Here's how the part is built. I have some questions about the finished solid (model axes, mm). A direction names the side the tool comes from. Coordinates: 2 decimals unless noted, no trailing zeros. Order: outer loops, then holes, each group sorted by start corner. A loop starts at its lowest first (then second) coordinate and runs counter-clockwise, first axis right, second up.
```python
from build123d import *

# Parameters (mm, degrees)
F0_W          = 155
F0_H          = 40
F0_R          = 5
F1_DEPTH      = 25
F2_R          = 11
F3_DEPTH      = 10
F4_W          = 40
F4_H          = 25
F5_DEPTH      = 25
F6_R          = 4.25
F7_DEPTH      = 40
F9_DEPTH      = 6
F10_T4_DEPTH  = 25
F10_T10_DEPTH = 25
F10_T16_DEPTH = 25
F10_T23_DEPTH = 25
F10_T29_DEPTH = 25
F10_T35_DEPTH = 25
F10_T41_DEPTH = 25
F10_T47_DEPTH = 25
F10_T54_DEPTH = 25
F10_T60_DEPTH = 25
F10_T63_DEPTH = 50


# Not quite as in the source:
# - a fillet or chamfer that OpenCascade refuses, or shapes differently, is made with other operations: its cross-section is extruded or revolved along the edge and cut away or added


with BuildPart() as f1:
    # F0 (on Front) → F1 (new body)
    with BuildSketch(Plane.XZ):
        with Locations((-7.5, 0)):
            Rectangle(F0_W, F0_H)
        with Locations((-65, 0)):
            Circle(F0_R, mode=Mode.SUBTRACT)
        Circle(F0_R, mode=Mode.SUBTRACT)
        with Locations((55, 0)):
            Circle(F0_R, mode=Mode.SUBTRACT)
    extrude(amount=F1_DEPTH)

    # F2 (on face) → F3 (cut)
    with BuildSketch(Plane.XZ.offset(25)):
        with Locations((-65, 0)):
            Circle(F2_R)
        Circle(F2_R)
        with Locations((55, 0)):
            Circle(F2_R)
    extrude(amount=-F3_DEPTH, mode=Mode.SUBTRACT)

    # F4 (on face) → F5 (join)
    with BuildSketch(Plane(origin=(0, 0, 0), x_dir=(-1, 0, 0), z_dir=(0, 1, 0))):
        with Locations((65, 32.5)):
            Rectangle(F4_W, F4_H)
        with Locations((65, -32.5)):
            Rectangle(F4_W, F4_H)
    extrude(amount=-F5_DEPTH)

    # F6 (on face) → F7 (cut, through all)
    with BuildSketch(Plane(origin=(-85, 0, 0), x_dir=(0, -1, 0), z_dir=(-1, 0, 0))):
        with Locations((12.5, 27.5)):
            Circle(F6_R)
        with Locations((12.5, -27.5)):
            Circle(F6_R)
    extrude(amount=-F7_DEPTH, mode=Mode.SUBTRACT)

    # F8 (on face) → F9 (cut)
    with BuildSketch(Plane.YZ.offset(-45)):
        Polygon((-8.4585481157, 34.5), (-16.5414518843, 34.5), (-20.5829037687, 27.5), (-16.5414518843, 20.5), (-8.4585481157, 20.5), (-4.4170962313, 27.5), align=None)
        Polygon((-8.4585481157, -20.5), (-16.5414518843, -20.5), (-20.5829037687, -27.5), (-16.5414518843, -34.5), (-8.4585481157, -34.5), (-4.4170962313, -27.5), align=None)
    extrude(amount=-F9_DEPTH, mode=Mode.SUBTRACT)

    # F10: fillet of radius 5 on 6 edges, made by hand


with BuildPart() as f10_tool2:
    # F10_s3 → F10_t4 (new body)
    with BuildSketch(Plane.XZ):
        with BuildLine():
            ThreePointArc((-40, 20), (-43.5355339059, 21.4644660941), (-45, 25))
            Line((-45, 25), (-45, 20))
            Line((-45, 20), (-40, 20))
        make_face()
    extrude(amount=F10_T4_DEPTH)

    split(bisect_by=Plane.XY.offset(20.5), keep=Keep.BOTTOM)

    split(bisect_by=Plane(origin=(0, -15.2206714755, 8.7876587737), x_dir=(1, 0, 0), z_dir=(0, 0.8660254038, -0.5)), keep=Keep.TOP)


with BuildPart() as f1_1:
    add(f1.part)

    # F10_t1: union F10_tool2
    add(f10_tool2.part)


with BuildPart() as f10_tool8:
    # F10_s9 → F10_t10 (new body)
    with BuildSketch(Plane.XZ):
        with BuildLine():
            ThreePointArc((-40, 20), (-43.5355339059, 21.4644660941), (-45, 25))
            Line((-45, 25), (-45, 20))
            Line((-45, 20), (-40, 20))
        make_face()
    extrude(amount=F10_T10_DEPTH)

    split(bisect_by=Plane.XY.offset(20.5), keep=Keep.TOP)

    split(bisect_by=Plane(origin=(0, -15.2206714755, 8.7876587737), x_dir=(1, 0, 0), z_dir=(0, 0.8660254038, -0.5)), keep=Keep.TOP)


with BuildPart() as f1_2:
    add(f1_1.part)

    # F10_t7: union F10_tool8
    add(f10_tool8.part)


with BuildPart() as f10_tool14:
    # F10_s15 → F10_t16 (new body)
    with BuildSketch(Plane.XZ):
        with BuildLine():
            ThreePointArc((-40, 20), (-43.5355339059, 21.4644660941), (-45, 25))
            Line((-45, 25), (-45, 20))
            Line((-45, 20), (-40, 20))
        make_face()
    extrude(amount=F10_T16_DEPTH)

    split(bisect_by=Plane(origin=(0, -3.5293285245, -2.0376587737), x_dir=(1, 0, 0), z_dir=(0, 0.8660254038, 0.5)), keep=Keep.TOP)

    split(bisect_by=Plane.XY.offset(20.5), keep=Keep.BOTTOM)

    split(bisect_by=Plane(origin=(0, -15.2206714755, 8.7876587737), x_dir=(1, 0, 0), z_dir=(0, -0.8660254038, 0.5)), keep=Keep.TOP)


with BuildPart() as f1_3:
    add(f1_2.part)

    # F10_t13: union F10_tool14
    add(f10_tool14.part)


with BuildPart() as f10_tool21:
    # F10_s22 → F10_t23 (new body)
    with BuildSketch(Plane.XZ):
        with BuildLine():
            ThreePointArc((-40, 20), (-43.5355339059, 21.4644660941), (-45, 25))
            Line((-45, 25), (-45, 20))
            Line((-45, 20), (-40, 20))
        make_face()
    extrude(amount=F10_T23_DEPTH)

    split(bisect_by=Plane(origin=(0, -3.5293285245, -2.0376587737), x_dir=(1, 0, 0), z_dir=(0, -0.8660254038, -0.5)), keep=Keep.TOP)

    split(bisect_by=Plane.XY.offset(20.5), keep=Keep.BOTTOM)


with BuildPart() as f1_4:
    add(f1_3.part)

    # F10_t20: union F10_tool21
    add(f10_tool21.part)


with BuildPart() as f10_tool27:
    # F10_s28 → F10_t29 (new body)
    with BuildSketch(Plane.XZ):
        with BuildLine():
            ThreePointArc((-40, 20), (-43.5355339059, 21.4644660941), (-45, 25))
            Line((-45, 25), (-45, 20))
            Line((-45, 20), (-40, 20))
        make_face()
    extrude(amount=F10_T29_DEPTH)

    split(bisect_by=Plane(origin=(0, -3.5293285245, -2.0376587737), x_dir=(1, 0, 0), z_dir=(0, -0.8660254038, -0.5)), keep=Keep.TOP)

    split(bisect_by=Plane.XY.offset(20.5), keep=Keep.TOP)


with BuildPart() as f1_5:
    add(f1_4.part)

    # F10_t26: union F10_tool27
    add(f10_tool27.part)


with BuildPart() as f10_tool33:
    # F10_s34 → F10_t35 (new body)
    with BuildSketch(Plane.XZ):
        with BuildLine():
            ThreePointArc((-40, -20), (-43.5355339059, -21.4644660941), (-45, -25))
            Line((-45, -25), (-45, -20))
            Line((-45, -20), (-40, -20))
        make_face()
    extrude(amount=F10_T35_DEPTH)

    split(bisect_by=Plane.XY.offset(-20.5), keep=Keep.TOP)

    split(bisect_by=Plane(origin=(0, -15.2206714755, -8.7876587737), x_dir=(1, 0, 0), z_dir=(0, 0.8660254038, 0.5)), keep=Keep.TOP)


with BuildPart() as f1_6:
    add(f1_5.part)

    # F10_t32: union F10_tool33
    add(f10_tool33.part)


with BuildPart() as f10_tool39:
    # F10_s40 → F10_t41 (new body)
    with BuildSketch(Plane.XZ):
        with BuildLine():
            ThreePointArc((-40, -20), (-43.5355339059, -21.4644660941), (-45, -25))
            Line((-45, -25), (-45, -20))
            Line((-45, -20), (-40, -20))
        make_face()
    extrude(amount=F10_T41_DEPTH)

    split(bisect_by=Plane.XY.offset(-20.5), keep=Keep.BOTTOM)

    split(bisect_by=Plane(origin=(0, -15.2206714755, -8.7876587737), x_dir=(1, 0, 0), z_dir=(0, 0.8660254038, 0.5)), keep=Keep.TOP)


with BuildPart() as f1_7:
    add(f1_6.part)

    # F10_t38: union F10_tool39
    add(f10_tool39.part)


with BuildPart() as f10_tool45:
    # F10_s46 → F10_t47 (new body)
    with BuildSketch(Plane.XZ):
        with BuildLine():
            ThreePointArc((-40, -20), (-43.5355339059, -21.4644660941), (-45, -25))
            Line((-45, -25), (-45, -20))
            Line((-45, -20), (-40, -20))
        make_face()
    extrude(amount=F10_T47_DEPTH)

    split(bisect_by=Plane.XY.offset(-20.5), keep=Keep.TOP)

    split(bisect_by=Plane(origin=(0, -3.5293285245, 2.0376587737), x_dir=(1, 0, 0), z_dir=(0, 0.8660254038, -0.5)), keep=Keep.TOP)

    split(bisect_by=Plane(origin=(0, -15.2206714755, -8.7876587737), x_dir=(1, 0, 0), z_dir=(0, -0.8660254038, -0.5)), keep=Keep.TOP)


with BuildPart() as f1_8:
    add(f1_7.part)

    # F10_t44: union F10_tool45
    add(f10_tool45.part)


with BuildPart() as f10_tool52:
    # F10_s53 → F10_t54 (new body)
    with BuildSketch(Plane.XZ):
        with BuildLine():
            ThreePointArc((-40, -20), (-43.5355339059, -21.4644660941), (-45, -25))
            Line((-45, -25), (-45, -20))
            Line((-45, -20), (-40, -20))
        make_face()
    extrude(amount=F10_T54_DEPTH)

    split(bisect_by=Plane.XY.offset(-20.5), keep=Keep.TOP)

    split(bisect_by=Plane(origin=(0, -3.5293285245, 2.0376587737), x_dir=(1, 0, 0), z_dir=(0, -0.8660254038, 0.5)), keep=Keep.TOP)


with BuildPart() as f1_9:
    add(f1_8.part)

    # F10_t51: union F10_tool52
    add(f10_tool52.part)


with BuildPart() as f10_tool58:
    # F10_s59 → F10_t60 (new body)
    with BuildSketch(Plane.XZ):
        with BuildLine():
            ThreePointArc((-40, -20), (-43.5355339059, -21.4644660941), (-45, -25))
            Line((-45, -25), (-45, -20))
            Line((-45, -20), (-40, -20))
        make_face()
    extrude(amount=F10_T60_DEPTH)

    split(bisect_by=Plane.XY.offset(-20.5), keep=Keep.BOTTOM)

    split(bisect_by=Plane(origin=(0, -3.5293285245, 2.0376587737), x_dir=(1, 0, 0), z_dir=(0, -0.8660254038, 0.5)), keep=Keep.TOP)


with BuildPart() as f1_10:
    add(f1_9.part)

    # F10_t57: union F10_tool58
    add(f10_tool58.part)

    # F10_s64 → F10_t63 (cut)
    with BuildSketch(Plane.XZ.offset(-12.5)):
        with BuildLine():
            ThreePointArc((-50, 45), (-46.4644660941, 43.5355339059), (-45, 40))
            Line((-45, 40), (-45, 45))
            Line((-45, 45), (-50, 45))
        make_face()
        with BuildLine():
            ThreePointArc((-45, -40), (-46.4644660941, -43.5355339059), (-50, -45))
            Line((-50, -45), (-45, -45))
            Line((-45, -45), (-45, -40))
        make_face()
        with BuildLine():
            ThreePointArc((70, -15), (68.5355339059, -18.5355339059), (65, -20))
            Line((65, -20), (70, -20))
            Line((70, -20), (70, -15))
        make_face()
        with BuildLine():
            ThreePointArc((70, 15), (68.5355339059, 18.5355339059), (65, 20))
            Line((65, 20), (70, 20))
            Line((70, 20), (70, 15))
        make_face()
    extrude(amount=F10_T63_DEPTH, mode=Mode.SUBTRACT)


solid = f1_10.part
```
Q1. If we section it at C-C on z = 0: Write out the boundary of the cut face in (x, y).
Q2. For faces 1 (the flat face through (12, -12, -20)), 2 (the flat face through (2, -15, -5)), 3 (the flat face through (-51, -9, -24)), which set-ups out of +Z, -Z, +X, -X, +Y, -Y let a thin tool reach every point of the face, with its end or its side?
Q3. Will these pins go through, and if not, where does the flat tip stop? pin 1 (10 mm diameter, centred on x = -28, y = -12, fed in from -Z); pin 2 (3 mm diameter, centred on y = -10.5, z = -28.5, fed in from -X); pin 3 (4 mm diameter, centred on x = -44.5, y = -11.5, fed in from +Z); pin 4 (12 mm diameter, centred on y = -14, z = -30, fed in from +X).
Q4. I need wall thicknesses on L1, parallel to Z at x = -65.5, y = -12.5; L2, parallel to X at y = -8, z = 0; L3, parallel to Z at x = 55, y = -10.25. Which ranges of each line are inside material? Lowest first, please.
Q5. If we section it at A-A on x = 0: Write out the boundary of the cut face in (y, z).
Q6. If we section it at D-D on x = -72: Write out the boundary of the cut face in (y, z), then the cut area to 3 significant figures.
Q7. We'd pull the mould along Z, two halves only. Please class faces 4 (the flat face through (-45, -12, -36)), 5 (the cylindrical face through (-46, -12, -43)), 6 (the flat face through (-51, -9, 31)), 7 (the cylindrical face through (69, -12, 18)): pulls with the +Z half, pulls with the -Z half, needs draft (parallel to the pull), parting line crosses it, or undercut.
Q8. If we section it at B-B on y = -12.5: Give the number of separate pieces and of enclosed holes in the cut face, then the cut area to 3 significant figures.
Reply:
1. outline: (-85, -25) - (-76, -25) - (-76, -15) - (-70, -15) - (-70, 0) - (-85, 0) - close; (-60, -15) - (-54, -15) - (-54, -25) - (-11, -25) - (-11, -15) - (-5, -15) - (-5, 0) - (-60, 0) - close; (5, -15) - (11, -15) - (11, -25) - (44, -25) - (44, -15) - (50, -15) - (50, 0) - (5, 0) - close; (60, -15) - (66, -15) - (66, -25) - (70, -25) - (70, 0) - (60, 0) - close
2. face 1: -Z, +X, +Y, -Y
2. face 2: -Y
2. face 3: +X
3. pin 1: stops at z = -20
3. pin 2: passes through
3. pin 3: stops at z = 43.57
3. pin 4: stops at x = -45
4. L1: z = -45 to -31.75, -23.25 to -4.97, 4.97 to 23.25, 31.75 to 45
4. L2: x = -85 to -70, -60 to -5, 5 to 50, 60 to 70
4. L3: z = -20 to -5, 5 to 20
5. outline: (-25, -20) - (0, -20) - (0, -5) - (-15, -5) - (-15, -11) - (-25, -11) - close; (-25, 11) - (-15, 11) - (-15, 5) - (0, 5) - (0, 20) - (-25, 20) - close
6. outline: (-25, -45) - (0, -45) - (0, 45) - (-25, 45) - (-25, 8.49) - (-15, 8.49) - (-15, -8.49) - (-25, -8.49) - close; hole circle Ø8.5 at (-12.5, -27.5); hole circle Ø8.5 at (-12.5, 27.5)
6. area: 1,970 mm2
7. face 4: needs draft
7. face 5: pulls with the -Z half
7. face 6: undercut
7. face 7: pulls with the +Z half
8. separate pieces: 3
8. enclosed holes: 3
8. area: 7,200 mm2
